Source: CAD feature listing. Evaluate the final solid. Frame: model axes, mm. A direction names the side the tool comes from. Coordinates: 2 decimals unless noted, no trailing zeros. Order: outer loops, then holes, each group sorted by start corner. A loop starts at its lowest first (then second) coordinate and runs counter-clockwise, first axis right, second up.
```python
from build123d import *

# Parameters (mm, degrees)
F0_R      = 7
F1_DEPTH  = 5
F2_R      = 4
F3_DEPTH  = 6
F4_R      = 1.2
F5_DEPTH  = 9
F6_R      = 5
F7_DEPTH  = 2
F8_R      = 6.5
F8_R_2    = 5.75
F9_DEPTH  = 0.5
F10_SIZE  = 0.2
F11_R     = 0.2
F13_R     = 1.25
F14_DEPTH = 4.5


with BuildPart() as f1:
    # F0 (on Top) → F1 (new body)
    with BuildSketch(Plane.XY):
        Circle(F0_R)
    extrude(amount=F1_DEPTH)

    # F2 (on face) → F3 (join)
    with BuildSketch(Plane(origin=(0, 0, 0), x_dir=(1, 0, 0), z_dir=(0, 0, -1))):
        Circle(F2_R)
    extrude(amount=F3_DEPTH)

    # F4 (on face) → F5 (cut)
    with BuildSketch(Plane(origin=(0, 0, -6), x_dir=(1, 0, 0), z_dir=(0, 0, -1))):
        Circle(F4_R)
    extrude(amount=-F5_DEPTH, mode=Mode.SUBTRACT)

    # F6 (on face) → F7 (cut)
    with BuildSketch(Plane.XY.offset(5)):
        Circle(F6_R)
    extrude(amount=-F7_DEPTH, mode=Mode.SUBTRACT)

    # F8 (on face) → F9 (cut)
    with BuildSketch(Plane.XY.offset(5)):
        Circle(F8_R)
        Circle(F8_R_2, mode=Mode.SUBTRACT)
    extrude(amount=-F9_DEPTH, mode=Mode.SUBTRACT)

    # F10
    f10_edges = [f1.edges().sort_by_distance(p)[0] for p in [
        (-5.75, 0, 5),
    ]]
    chamfer(f10_edges, length=F10_SIZE)

    # F11
    f11_edges = [f1.edges().sort_by_distance(p)[0] for p in [
        (-5.75, 0, 4.8),
        (-1.2, 0, 3),
        (-1.2, 0, -6),
    ]]
    fillet(f11_edges, radius=F11_R)

    # F13 (on Right) → F14 (cut)
    with BuildSketch(Plane.YZ):
        with Locations((0, -3.5)):
            Circle(F13_R)
    extrude(amount=-F14_DEPTH, mode=Mode.SUBTRACT)


solid = f1.part
```
1. Section query D-D, the plane z = -3.5. Output: boundary loops of the cut face in (x, y).
2. Section query A-A, the plane z = 2. Output: boundary loops of the cut face in (x, y), plus the area to 3 significant figures.
3. Section query C-C, the plane x = -6. Output: boundary loops of the cut face in (y, z), plus the area to 3 significant figures.
4. Access query for faces 4 (the flat face through (3, -3, 0)), 5 (the flat face through (-1.2, -1, 3)), 6 (the cylindrical face through (-2.42, 1.19, -3.12)). Directions: +Z, -Z, +X, -X, +Y, -Y. A direction counts if a zero-diameter tool reaches every point of the face in a straight line with its end or side. Return the directions, or none.
5. Section query B-B, the plane y = 0. Count the separate pieces of the cut face and the enclosed holes in it, plus the area to 3 significant figures.
6. Material intervals for line 1 along Y through (x, z) = (0, -1.75); line 2 along Z through (x, y) = (-2.35, 0); line 3 along X through (y, z) = (0, -3), sorted ascending.
7. Contact query for flat-ended pins moving along their axis: P1, Ø6, axis at x = 0, y = 0, coming from the +Z side; P2, Ø3, axis at y = 0, z = -3.5, coming from the -X side; P3, Ø2, axis at x = -5, z = -4.5, coming from the -Y side. Output: stop coordinate, or through.
8. Draft query along X for faces 1 (the flat face through (-5, 2, 5)), 2 (the cylindrical face through (-5.158, -3.955, 4.754)), 3 (the cylindrical face through (6.466, -2.681, 2.465)). Return one class per face: +X half, -X half, draft (parallel to the pull), parting line (faces both ways), or undercut.
Answer key:
1. outline: (-3.8, -1.25) arc R4 ccw (long way) to (-3.8, 1.25) - (0, 1.25) - (0, 1.2) arc R1.2 cw to (0, -1.2) - (0, -1.25) - close
2. outline: circle Ø14 at (0, 0); hole circle Ø2.4 at (0, 0)
2. area: 149 mm2
3. outline: (-3.61, 0) - (3.61, 0) - (3.61, 5) - (2.5, 5) - (2.5, 4.5) - (-2.5, 4.5) - (-2.5, 5) - (-3.61, 5) - close
3. area: 33.6 mm2
4. face 4: -Z
4. face 5: +Z
4. face 6: -X
5. separate pieces: 3
5. enclosed holes: 0
5. area: 68.6 mm2
6. line 1: y = -4 to -1.2, 1.2 to 4
6. line 2: z = -6 to -4.75, -2.25 to 3
6. line 3: x = 1.2 to 4
7. P1: stops at z = 3
7. P2: stops at x = -4
7. P3: passes through
8. face 1: draft
8. face 2: undercut
8. face 3: parting line
